```python
from build123d import *

# Parameters (mm, degrees)
F0_R     = 45.231736
F1_DEPTH = 63.5
F2_R     = 16.885337
F2_R_2   = 17.383209
F3_DEPTH = 12.7


with BuildPart() as f1:
    # F0 (on Front) → F1 (new body)
    with BuildSketch(Plane.XZ):
        Circle(F0_R)
    extrude(amount=F1_DEPTH)

    # F2 (on Front) → F3 (join)
    with BuildSketch(Plane.XZ):
        with Locations((-26.454598, 48.025273)):
            Circle(F2_R)
        with Locations((33.983976, 45.176312)):
            Circle(F2_R_2)
    extrude(amount=F3_DEPTH)


solid = f1.part
```
Can you work these out from the model? Positions are in its coordinate system, mm. A direction names the side the tool comes from. Round coordinates to 2 decimals unless told otherwise and drop trailing zeros. Loops run counter-clockwise (first coordinate to the right, second up) from the corner with the lowest first, then second, coordinate; pieces in that order, holes last.
Item 1: Suppose I cut it at B-B, the plane x = 32.5. Write out the boundary of the cut face in (y, z), then the cut area to 3 significant figures.
Item 2: Which directions (+Z, -Z, +X, -X, +Y, -Y) give clear straight access to the entire face, cutting with the end or side of a thin tool? Please do faces 3 (the flat face through (34, -12.7, 45)), 4 (the flat face through (-27, -12.7, 49)), 5 (the flat face through (2, 0, 11)).
Item 3: Suppose I cut it at D-D, the plane x = 0. Write out the boundary of the cut face in (y, z), then the cut area to 3 significant figures.
Item 4: Will these pins go through, and if not, where does the flat tip stop? pin 1 Ø2 at (x, y) = (2, -56) entering from -Z; pin 2 Ø3 at (x, y) = (-9, -26.5) entering from -Z; pin 3 Ø1.5 at (x, y) = (-24.5, -26) entering from +Z; pin 4 Ø6 at (x, z) = (35.5, 50) entering from +Y.
Item 5: If we mould it in two halves opening along X, with no side actions, what happens to faces 1 (the cylindrical face through (44.895, -6.261, 58.709)), 2 (the flat face through (-1, -63.5, 1))? For each: +X half, -X half, draft (parallel to the pull), parting line (faces both ways), or undercut.
Item 6: Please list where these lines run through material, in increasing order: L1, parallel to X at y = -8, z = 54.5; L2, parallel to Z at x = 25, y = -5; L3, parallel to X at y = -26.5, z = 8.
Item 7: Suppose I cut it at A-A, the plane y = -30. Write out the boundary of the cut face in (x, z), then the cut area to 3 significant figures.
Item 8: Suppose I cut it at C-C, the plane z = 0. Write out the boundary of the cut face in (x, y).
Reported:
1. outline: (-63.5, -31.46) - (0, -31.46) - (0, 62.5) - (-12.7, 62.5) - (-12.7, 31.46) - (-63.5, 31.46) - close
1. area: 4,390 mm2
2. face 3: +Z, +X, -Y
2. face 4: +Z, -X, -Y
2. face 5: +Z, -Z, +X, -X, +Y
3. outline: (-63.5, -45.23) - (0, -45.23) - (0, 45.23) - (-63.5, 45.23) - close
3. area: 5,740 mm2
4. pin 1: stops at z = -45.22
4. pin 2: stops at z = -44.61
4. pin 3: stops at z = 38.49
4. pin 4: stops at y = 0
5. face 1: undercut
5. face 2: draft
6. L1: x = -42.05 to -10.86, 19.31 to 48.66
6. L2: z = -37.69 to 60.06
6. L3: x = -44.52 to 44.52
7. outline: circle Ø90.46 at (0, 0)
7. area: 6,430 mm2
8. outline: (-45.23, -63.5) - (45.23, -63.5) - (45.23, 0) - (-45.23, 0) - close
